Input: part model. Units: mm. Frame: model coordinates. A direction names the side the tool comes from. Give positions to 0.01 mm unless a question says otherwise; leave off trailing zeros. Write each loop counter-clockwise with the first axis right and the second up, starting at its lowest first coordinate (ties: lowest second). Pieces come first, ordered by that corner, then holes.
```python
from build123d import *

# Parameters (mm, degrees)
SKETCH_1_W           = 3.5
SKETCH_1_H           = 9.2
EXTRUDE_1_DEPTH      = 7.2
SKETCH_2_W           = 2.75
SKETCH_2_H           = 3.05
CUT_EXTRUDE_1_DEPTH  = 0.4
SKETCH_5_W           = 2.75
SKETCH_5_H           = 3.8
CUT_EXTRUDE_4_DEPTH  = 0.4
CUT_EXTRUDE_6_REACH  = 10.533
SKETCH_9_R           = 0.9
EXTRUDE_3_DEPTH      = 1.3
SKETCH_10_W          = 0.8
SKETCH_10_H          = 3
CUT_EXTRUDE_7_DEPTH  = 1.2
SKETCH_11_W          = 0.8
SKETCH_11_H          = 2
CUT_EXTRUDE_8_DEPTH  = 0.8
FILLET_2_R           = 0.2
CUT_EXTRUDE_12_REACH = 11.445
DRAFT_3_ANGLE        = -25.463345062
DRAFT_4_ANGLE        = -25.463345062
CUT_EXTRUDE_15_REACH = 11.445
SKETCH_18_W          = 0.4
SKETCH_18_H          = 1.9
CUT_EXTRUDE_16_REACH = 11.445
SKETCH_19_W          = 0.4
SKETCH_19_H          = 1.9


with BuildPart() as part:
    # Эскиз1 → Бобышка-Вытянуть1 (new body)
    with BuildSketch(Plane.XZ.offset(3.6)):
        with Locations((-1.75, 0)):
            Rectangle(SKETCH_1_W, SKETCH_1_H)
    extrude(amount=-EXTRUDE_1_DEPTH)

    # Эскиз2 → Вырез-Вытянуть1 (cut)
    with BuildSketch(Plane.XZ.offset(3.6)):
        with Locations((-1.75, -3.075)):
            Rectangle(SKETCH_2_W, SKETCH_2_H)
    extrude(amount=-CUT_EXTRUDE_1_DEPTH, mode=Mode.SUBTRACT)

    # Эскиз5 → Вырез-Вытянуть4 (cut)
    with BuildSketch(Plane(origin=(0, 0, -4.6), x_dir=(-1, 0, 0), z_dir=(0, 0, -1))):
        with Locations((1.75, -1.3)):
            Rectangle(SKETCH_5_W, SKETCH_5_H)
    extrude(amount=-CUT_EXTRUDE_4_DEPTH, mode=Mode.SUBTRACT)

    # Эскиз7 → Вырез-Вытянуть6 (cut, up to next)
    with BuildSketch(Plane(origin=(0, 0, -2.3), x_dir=(-1, 0, 0), z_dir=(0, 0, -1)), mode=Mode.PRIVATE) as cut_extrude_6_sk1:
        with BuildLine():
            Line((3.3, -1.1), (3.3, -0.1))
            Line((3.3, -0.1), (2.9, -0.1))
            Line((2.9, -0.1), (2.9, 1.1))
            Line((2.9, 1.1), (0.6, 1.1))
            Line((0.6, 1.1), (0.6, -0.1))
            Line((0.6, -0.1), (0.2, -0.1))
            Line((0.2, -0.1), (0.2, -1.1))
            Line((0.2, -1.1), (0.6, -1.1))
            Line((0.6, -1.1), (0.6, -3))
            ThreePointArc((0.6, -3), (1.75, -2.8), (2.9, -3))
            Line((2.9, -3), (2.9, -1.1))
            Line((2.9, -1.1), (3.3, -1.1))
        make_face()
    cut_extrude_6_tool1 = extrude(cut_extrude_6_sk1.sketch, amount=-CUT_EXTRUDE_6_REACH, mode=Mode.PRIVATE) & part.part
    add(cut_extrude_6_tool1.solids().sort_by_distance((-1.75, -0.860527, -2.3))[0], mode=Mode.SUBTRACT)

    # Эскиз9 → Бобышка-Вытянуть3 (add)
    with BuildSketch(Plane.XY.offset(-1)):
        with Locations((-1.75, -0.6)):
            Circle(SKETCH_9_R)
    extrude(amount=-EXTRUDE_3_DEPTH)

    # Эскиз10 → Вырез-Вытянуть7 (cut)
    with BuildSketch(Plane(origin=(0, 0, -4.2), x_dir=(-1, 0, 0), z_dir=(0, 0, -1))):
        with Locations((1.75, -1.7)):
            Rectangle(SKETCH_10_W, SKETCH_10_H)
    extrude(amount=-CUT_EXTRUDE_7_DEPTH, mode=Mode.SUBTRACT)

    # Эскиз11 → Вырез-Вытянуть8 (cut)
    with BuildSketch(Plane(origin=(0, -0.2, 0), x_dir=(1, 0, 0), z_dir=(0, 1, 0))):
        with Locations((-1.75, 2)):
            Rectangle(SKETCH_11_W, SKETCH_11_H)
    extrude(amount=-CUT_EXTRUDE_8_DEPTH, mode=Mode.SUBTRACT)

    # Скругление2
    fillet_2_edges = [part.edges().sort_by_distance(p)[0] for p in [
        (-2.65, -0.6, -1),
    ]]
    fillet(fillet_2_edges, radius=FILLET_2_R)

    # Эскиз15 → Вырез-Вытянуть12 (cut, up to next)
    with BuildSketch(Plane(origin=(0, 0, -3.4), x_dir=(-1, 0, 0), z_dir=(0, 0, -1)), mode=Mode.PRIVATE) as cut_extrude_12_sk1:
        Polygon((1.05, 2.05), (1.05, 1.45), (0.2, 1.45), (0.2, -0.1), (0.6, -0.1), (0.6, 1.1), (2.9, 1.1), (2.9, -0.1), (3.3, -0.1), (3.3, 1.45), (2.45, 1.45), (2.45, 2.05), (3.3, 2.05), (3.3, 3.1), (0.2, 3.1), (0.2, 2.05), align=None)
    cut_extrude_12_tool1 = extrude(cut_extrude_12_sk1.sketch, amount=-CUT_EXTRUDE_12_REACH, mode=Mode.PRIVATE) & part.part
    add(cut_extrude_12_tool1.solids().sort_by_distance((-1.75, 1.90798, -3.4))[0], mode=Mode.SUBTRACT)

    # Уклон3
    draft_3_faces = [part.faces().sort_by_distance(p)[0] for p in [
        (-0.2, 2.575, 0.6),
    ]]
    draft(draft_3_faces, Plane(origin=(-3.3, 3.1, 4.601), x_dir=(0, 0, -1), z_dir=(0, -1, 0)), DRAFT_3_ANGLE)

    # Уклон4
    draft_4_faces = [part.faces().sort_by_distance(p)[0] for p in [
        (-3.3, 2.575, 0.6),
    ]]
    draft(draft_4_faces, Plane(origin=(-3.3, 3.1, 4.601), x_dir=(0, 0, -1), z_dir=(0, -1, 0)), DRAFT_4_ANGLE)

    # Эскиз18 → Вырез-Вытянуть15 (cut, up to next)
    with BuildSketch(Plane(origin=(0, 0, -3.4), x_dir=(-1, 0, 0), z_dir=(0, 0, -1)), mode=Mode.PRIVATE) as cut_extrude_15_sk1:
        with Locations((0.4, -2.05)):
            Rectangle(SKETCH_18_W, SKETCH_18_H)
    cut_extrude_15_tool1 = extrude(cut_extrude_15_sk1.sketch, amount=-CUT_EXTRUDE_15_REACH, mode=Mode.PRIVATE) & part.part
    add(cut_extrude_15_tool1.solids().sort_by_distance((-0.4, -2.05, -3.4))[0], mode=Mode.SUBTRACT)

    # Эскиз19 → Вырез-Вытянуть16 (cut, up to next)
    with BuildSketch(Plane(origin=(0, 0, -3.4), x_dir=(-1, 0, 0), z_dir=(0, 0, -1)), mode=Mode.PRIVATE) as cut_extrude_16_sk1:
        with Locations((3.1, -2.05)):
            Rectangle(SKETCH_19_W, SKETCH_19_H)
    cut_extrude_16_tool1 = extrude(cut_extrude_16_sk1.sketch, amount=-CUT_EXTRUDE_16_REACH, mode=Mode.PRIVATE) & part.part
    add(cut_extrude_16_tool1.solids().sort_by_distance((-3.1, -2.05, -3.4))[0], mode=Mode.SUBTRACT)


solid = part.part
```
Q1. Section D-D, the plane z = -2.75. Give the number of separate pieces and of enclosed holes in the cut face, then the cut area to 3 significant figures.
Q2. Section A-A, the plane y = -0.6. Return the cut outline in (x, z) (3 decimals).
Q3. Section C-C, the plane x = -1.75. Return the cut outline in (y, z).
Q4. Access query for faces 1 (the flat face through (-2.15, -1.4, -3.3)), 2 (the flat face through (-2.9, -2, -3)), 3 (the flat face through (-2, 3.6, 0)). Directions: +Z, -Z, +X, -X, +Y, -Y. A direction counts if a zero-diameter tool reaches every point of the face in a straight line with its end or side. Return the directions, or none.
Q5. Material intervals for line 1 along Y through (x, z) = (-1.8, -2.25); line 2 along Y through (x, z) = (-0.8, -3.25); line 3 along Y through (x, z) = (-1.65, -2.5), sorted ascending.
Q6. Section B-B, the plane z = 0. Return the cut outline in (x, y), then the cut area to 3 significant figures.
Q7. Mould query, pull axis X, two halves, no side actions, for faces 4 (the flat face through (-0.2, -1, 1)), 5 (the flat face through (-3.5, 0, 0)), 6 (the flat face through (-2, -3.6, 1)). Classes: +X half, -X half, draft (parallel to the pull), parting line (faces both ways), or undercut.
Solutions:
1. separate pieces: 1
1. enclosed holes: 4
1. area: 16.3 mm2
2. outline: (-3.5, -4.6) - (-3.125, -4.6) - (-3.125, -4.2) - (-2.15, -4.2) - (-2.15, -1) - (-2.45, -1) arc R0.2 ccw to (-2.65, -1.2) - (-2.65, -2.3) - (-3.3, -2.3) - (-3.3, 4.6) - (-3.5, 4.6) - close; (-1.35, -4.2) - (-0.375, -4.2) - (-0.375, -4.6) - (0, -4.6) - (0, 4.6) - (-0.2, 4.6) - (-0.2, -2.3) - (-0.85, -2.3) - (-0.85, -1.2) arc R0.2 ccw to (-1.05, -1) - (-1.35, -1) - close
3. outline: (-3.6, -1.55) - (-3.2, -1.55) - (-3.2, -3) - (-1, -3) - (-1, -1) - (-1.3, -1) arc R0.2 ccw to (-1.5, -1.2) - (-1.5, -2.3) - (-2.8, -2.3) - (-2.8, 4.6) - (-3.6, 4.6) - close; (-0.2, -4.2) - (0.6, -4.2) - (0.6, -4.6) - (3.6, -4.6) - (3.6, 4.6) - (3.1, 4.6) - (3.1, -3.4) - (1.1, -3.4) - (1.1, -2.3) - (0.3, -2.3) - (0.3, -1.2) arc R0.2 ccw to (0.1, -1) - (-0.2, -1) - close
4. face 1: -Z
4. face 2: +Z
4. face 3: +Z, -Z, +X, -X, +Y
5. line 1: y = -3.2 to -2.8, -1.5 to -1, -0.2 to 0.3, 3.1 to 3.6
5. line 2: y = -3.2 to 1.1, 1.45 to 2.05, 3.1 to 3.6
5. line 3: y = -3.2 to -1, -0.2 to 1.1, 3.1 to 3.6
6. outline: (-3.5, -3.6) - (0, -3.6) - (0, 3.6) - (-3.5, 3.6) - close; hole (-3.3, -3) - (-2.9, -3) arc R3.41 cw to (-0.6, -3) - (-0.2, -3) - (-0.2, 1.45) - (-1.05, 1.45) - (-1.05, 2.05) - (-0.7, 2.05) - (-0.2, 3.1) - (-3.3, 3.1) - (-2.8, 2.05) - (-2.45, 2.05) - (-2.45, 1.45) - (-3.3, 1.45) - close
6. area: 8.14 mm2
7. face 4: undercut
7. face 5: -X half
7. face 6: draft
